```python
from build123d import *

# Parameters (mm, degrees)
F1_DEPTH = 939.8
F2_R     = 2.6162
F3_DEPTH = 50.801


with BuildPart() as f1:
    # F0 (on Right) → F1 (new body)
    with BuildSketch(Plane.YZ):
        with BuildLine():
            Line((0, -44.45), (0, 0))
            Line((0, 0), (-3.175, 0))
            Line((-3.175, 0), (-3.175, -50.8))
            Line((-3.175, -50.8), (47.625, -50.8))
            Line((47.625, -50.8), (47.625, -47.625))
            Line((47.625, -47.625), (3.175, -47.625))
            ThreePointArc((3.175, -47.625), (0.929936, -46.695064), (0, -44.45))
        make_face()
    extrude(amount=-F1_DEPTH)

    # F2 (on face) → F3 (cut, through all)
    with BuildSketch(Plane.XZ.offset(3.175)):
        with Locations((-14.2875, -40.7416)):
            Circle(F2_R)
        with Locations((-14.2875, -10.0584)):
            Circle(F2_R)
        with Locations((-925.5125, -40.7416)):
            Circle(F2_R)
        with Locations((-925.5125, -10.0584)):
            Circle(F2_R)
        with Locations((-431.8, -10.0584)):
            Circle(F2_R)
        with Locations((-431.8, -40.7416)):
            Circle(F2_R)
        with Locations((-64.77, -25.4)):
            Circle(F2_R)
        with Locations((-762, -25.4)):
            Circle(F2_R)
        with Locations((-900.1125, -10.0584)):
            Circle(F2_R)
        with Locations((-900.1125, -40.7416)):
            Circle(F2_R)
        with Locations((-39.6875, -10.0584)):
            Circle(F2_R)
        with Locations((-39.6875, -40.7416)):
            Circle(F2_R)
        with Locations((-859.9678, -10.0584)):
            Circle(F2_R)
        with Locations((-859.9678, -40.7416)):
            Circle(F2_R)
        with Locations((-731.8, -10.0584)):
            Circle(F2_R)
        with Locations((-731.8, -40.7416)):
            Circle(F2_R)
        with Locations((-581.8, -10.0584)):
            Circle(F2_R)
        with Locations((-581.8, -40.7416)):
            Circle(F2_R)
        with Locations((-281.8, -10.0584)):
            Circle(F2_R)
        with Locations((-281.8, -40.7416)):
            Circle(F2_R)
        with Locations((-131.8, -10.0584)):
            Circle(F2_R)
        with Locations((-131.8, -40.7416)):
            Circle(F2_R)
    extrude(amount=-F3_DEPTH, mode=Mode.SUBTRACT)


solid = f1.part
```
For this review, take the finished solid that the model builds, in its own axes (mm). A direction names the side the tool comes from. Round coordinates to 2 decimals unless told otherwise and drop trailing zeros. Write each loop counter-clockwise with the first axis right and the second up, starting at its lowest first coordinate (ties: lowest second). Pieces come first, ordered by that corner, then holes. Notation, with made-up numbers: M 78.25,4 L 137.25,4 A24 cw 137.25,32 Z; hole C 83,19 d6. An arc over 180 degrees is marked long. One line per item, written item: value. Start each with the question number.
(1) Wall thickness on line 1 (Z direction, x = -131.8, y = -2.45); line 2 (Z direction, x = -731, y = -1); line 3 (Z direction, x = -762, y = -1): over which ranges is each line inside the solid? List them lowest first.
(2) Insertion check: pin 1 (3 mm diameter, centred on x = -277.5, z = -32, fed in from +Y); pin 2 (5 mm diameter, centred on x = -828, y = 36, fed in from +Z) (3 decimals); pin 3 (8.5 mm diameter, centred on x = -39.69, z = -10.06, fed in from -Y) (3 decimals). Each pin has a flat end and moves straight along its axis. Give the tip position at first contact, or say it passes through.
(3) We need section B-B (y = 25). Give the boundary of the cut face in (x, z) (3 decimals), and give its area (3 significant figures).
(4) We need section A-A (x = -555). Give the boundary of the cut face in (y, z) (3 decimals).
(5) Machinability: for faces 1 (the flat face through (-463, 26, -47.625)), 2 (the flat face through (-463, -3.175, -25)), which of the approach directions +Z, -Z, +X, -X, +Y, -Y give a long, thin tool a straight path to every point of the face, cutting with its end or side? Answer none if there is none.
Result:
1. line 1: -50.8 to -43.36, -38.13 to -12.67, -7.44 to 0
1. line 2: -50.8 to -43.23, -38.25 to -12.55, -7.57 to 0
1. line 3: -50.8 to -28.02, -22.78 to 0
2. pin 1: y = 0
2. pin 2: z = -47.625
2. pin 3: y = -3.175
3. outline: M -939.8,-50.8 L 0,-50.8 L 0,-47.625 L -939.8,-47.625 Z
3. area: 2,980 mm²
4. outline: M -3.175,-50.8 L 47.625,-50.8 L 47.625,-47.625 L 3.175,-47.625 A3.175 cw 0,-44.45 L 0,0 L -3.175,0 Z
5. face 1: +Z, +X, -X, +Y
5. face 2: +Z, -Z, +X, -X, -Y
